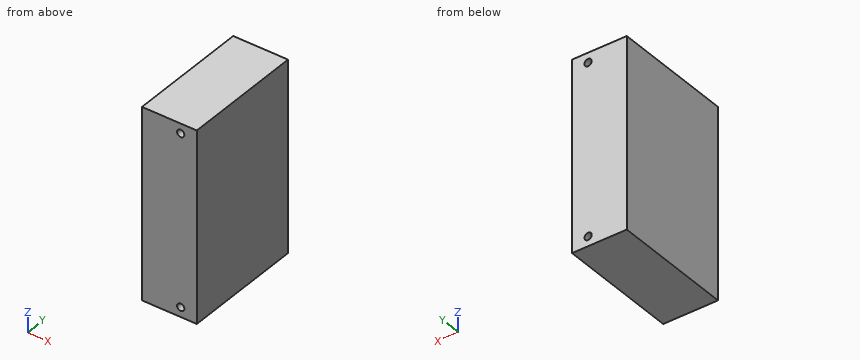
from build123d import *

# Parameters (mm, degrees)
SKETCH_1_W          = 34
SKETCH_1_H          = 118
EXTRUDE_1_DEPTH     = 76
SKETCH_2_R          = 2.25
CUT_EXTRUDE_1_DEPTH = 98.703633505


with BuildPart() as part:
    # 草图1 → 凸台-拉伸1 (new body)
    with BuildSketch(Plane(origin=(0, 0, 0), x_dir=(1, 0, 0), z_dir=(0, 1, 0))):
        Rectangle(SKETCH_1_W, SKETCH_1_H)
    extrude(amount=EXTRUDE_1_DEPTH)

    # 草图2 → 切除-拉伸1 (cut, through all)
    with BuildSketch(Plane.XZ):
        with Locations(Location((7, 53, 0), (0, 0, 270))):
            Circle(SKETCH_2_R)
        with Locations(Location((7, -53, 0), (0, 0, 90))):
            Circle(SKETCH_2_R)
    extrude(amount=-CUT_EXTRUDE_1_DEPTH, mode=Mode.SUBTRACT)


solid = part.part
Verification items for the finished model (mm, model axes). Give positions to 0.01 mm unless a question says otherwise; leave off trailing zeros. Write each loop counter-clockwise with the first axis right and the second up, starting at its lowest first coordinate (ties: lowest second). Pieces come first, ordered by that corner, then holes.
(1) Cross-section at B-B (x = 7). Enter the section's corners in (y, z).
(2) Cross-section at A-A (z = 53). Enter the section's corners in (x, y).
(3) Material ranges on line 1 (Z direction, x = 8, y = 59); line 2 (X direction, y = 45, z = 53); line 3 (Z direction, x = 5.5, y = 64), recorded low to high.
Worked out:
1. outline: (0, -59) - (76, -59) - (76, -55.25) - (0, -55.25) - close; (0, -50.75) - (76, -50.75) - (76, 50.75) - (0, 50.75) - close; (0, 55.25) - (76, 55.25) - (76, 59) - (0, 59) - close
2. outline: (-17, 0) - (4.75, 0) - (4.75, 76) - (-17, 76) - close; (9.25, 0) - (17, 0) - (17, 76) - (9.25, 76) - close
3. line 1: z = -59 to -55.02, -50.98 to 50.98, 55.02 to 59
3. line 2: x = -17 to 4.75, 9.25 to 17
3. line 3: z = -59 to -54.68, -51.32 to 51.32, 54.68 to 59
